The figure shows three views and two pictorial views of one solid part (mm, origin at its lowest corner). Answer the questions. A direction names the side the tool comes from. Give positions to 0.01 mm unless a question says otherwise; leave off trailing zeros. Order: outer loops, then holes, each group sorted by start corner. A loop starts at its lowest first (then second) coordinate and runs counter-clockwise, first axis right, second up. Notation, with made-up numbers: (-4.75, -28.75) -> (42.25, -28.75) arc R19 cw to (42.25, -6.75) -> close; hole circle Ø7 at (-13.5, -12). An arc over 180 degrees is marked (long way). Use one line per item in the form item = value.
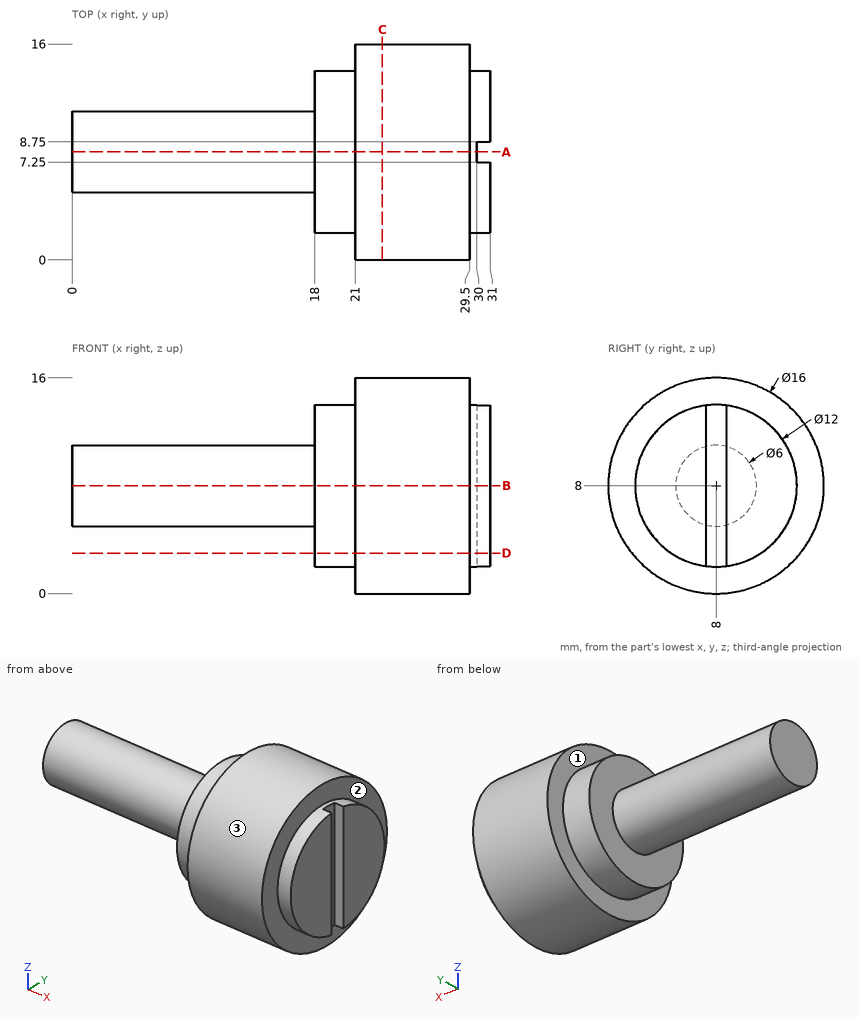
Item 1: Which of the six approach directions +Z, -Z, +X, -X, +Y, -Y give full straight-line access (tool end or side, diameter ignored) to the marked faces 1, 2 and 3?
Checks:
face_1 = -X
face_2 = +X
face_3 = +X, -X
Item 2: Given pin 1 Ø9.5 at (y, z) = (9.5, 9) entering from -X; pin 2 Ø3 at (x, y) = (13.5, 5.5) entering from -Z; pin 3 Ø0.8 at (x, z) = (30.5, 7) entering from -Y; pin 4 Ø1 at (y, z) = (13, 11.5) entering from -X, each flat-ended and moving along its own axis, determine where each tip first touches the part or whether it passes through.
Checks:
pin_1 = 0
pin_2 = 5.17
pin_3 = 2.03
pin_4 = 18
Item 3: The part is cut by section C-C on x = 23. Give the vertices of the cut face in (y, z).
Checks:
outline = circle Ø16 at (8, 8)
Item 4: The part is cut by section A-A on y = 8. Give the vertices of the cut face in (x, z), and give its area (3 significant figures).
Checks:
outline = (0, 5) -> (18, 5) -> (18, 2) -> (21, 2) -> (21, 0) -> (29.5, 0) -> (29.5, 2) -> (30, 2) -> (30, 14) -> (29.5, 14) -> (29.5, 16) -> (21, 16) -> (21, 14) -> (18, 14) -> (18, 11) -> (0, 11) -> close
area = 286 mm²
Item 5: Straight lines are drawn through the part: L1, parallel to X at y = 9.5, z = 13; L2, parallel to X at y = 1.25, z = 5.75; L3, parallel to Y at x = 1, z = 10.75. For each, find the intervals that lie inside material, in ascending order. Write a range as from..to.
Checks:
L1 = 18..31
L2 = 21..29.5
L3 = 6.8..9.2
Item 6: The part is cut by section B-B on z = 8. Give the vertices of the cut face in (x, y).
Checks:
outline = (0, 5) -> (18, 5) -> (18, 2) -> (21, 2) -> (21, 0) -> (29.5, 0) -> (29.5, 2) -> (31, 2) -> (31, 7.25) -> (30, 7.25) -> (30, 8.75) -> (31, 8.75) -> (31, 14) -> (29.5, 14) -> (29.5, 16) -> (21, 16) -> (21, 14) -> (18, 14) -> (18, 11) -> (0, 11) -> close
Item 7: The part is cut by section D-D on z = 3. Give the vertices of the cut face in (x, y) (3 decimals).
Checks:
outline = (18, 4.683) -> (21, 4.683) -> (21, 1.755) -> (29.5, 1.755) -> (29.5, 4.683) -> (31, 4.683) -> (31, 7.25) -> (30, 7.25) -> (30, 8.75) -> (31, 8.75) -> (31, 11.317) -> (29.5, 11.317) -> (29.5, 14.245) -> (21, 14.245) -> (21, 11.317) -> (18, 11.317) -> close
